Input: dimensioned drawing with shaded views. Units: mm. Origin: part minimum x, y, z. Coordinates: 2 decimals unless noted, no trailing zeros. Order: outer loops, then holes, each group sorted by start corner. A loop starts at its lowest first (then second) coordinate and runs counter-clockwise, first axis right, second up. Notation, with made-up numbers: (50, 18) - (80, 18) arc R27 cw to (80, 41) - close; hole circle Ø1 at (44.5, 29). An arc over 180 degrees is marked (long way). One line per question, with ' | ' between items. Start each with the question number.
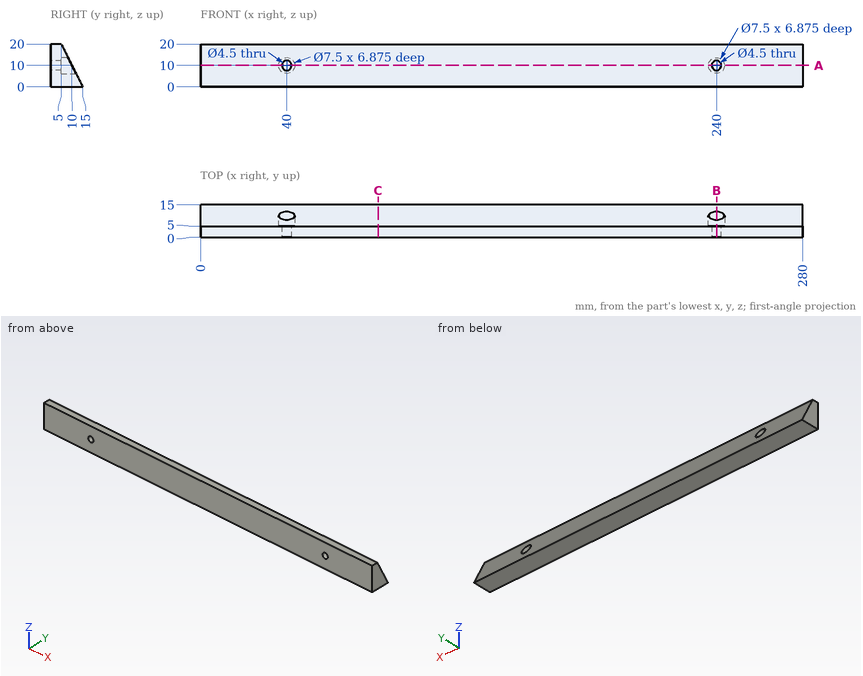
(1) Material intervals for line 1 along X through (y, z) = (7.25, 13); line 2 along Z through (x, y) = (240, 1.8); line 3 along X through (y, z) = (8, 8.5), sorted ascending. Write a range as from..to.
(2) Pin query (flat end, axial travel): pin 1 (8 mm diameter, centred on x = 41, z = 12, fed in from +Y); pin 2 (1.5 mm diameter, centred on y = 10.5, z = 14.5, fed in from +X) (1 decimal); pin 3 (8 mm diameter, centred on x = 240, z = 10, fed in from +Y); pin 4 (8.5 mm diameter, centred on x = 40, z = 10, fed in from +Y) (3 decimals). Return the tip coordinate at first contact, or that it passes through.
(3) Section A-A (z = 10). Output: boundary loops of the cut face in (x, y), then the cut area to 3 significant figures.
(4) Section B-B (x = 240). Output: boundary loops of the cut face in (y, z) (3 decimals).
(5) Section C-C (x = 82.5). Output: boundary loops of the cut face in (y, z), then the cut area to 3 significant figures.
Worked answers:
1) line 1: x = 0..37.75, 42.25..237.75, 242.25..280 | line 2: z = 0..7.75, 12.25..20 | line 3: x = 0..36.56, 43.44..236.56, 243.44..280
2) pin 1: stops at y = 10.52 | pin 2: passes through | pin 3: stops at y = 12 | pin 4: stops at y = 12.125
3) outline: (0, 0) - (37.75, 0) - (37.75, 5) - (36.25, 5) - (36.25, 10) - (0, 10) - close; (42.25, 0) - (237.75, 0) - (237.75, 5) - (236.25, 5) - (236.25, 10) - (43.75, 10) - (43.75, 5) - (42.25, 5) - close; (242.25, 0) - (280, 0) - (280, 10) - (243.75, 10) - (243.75, 5) - (242.25, 5) - close | area: 2,680 mm²
4) outline: (0, 0) - (15, 0) - (11.875, 6.25) - (5, 6.25) - (5, 7.75) - (0, 7.75) - close; (0, 12.25) - (5, 12.25) - (5, 13.75) - (8.125, 13.75) - (5, 20) - (0, 20) - close
5) outline: (0, 0) - (15, 0) - (5, 20) - (0, 20) - close | area: 200 mm²
